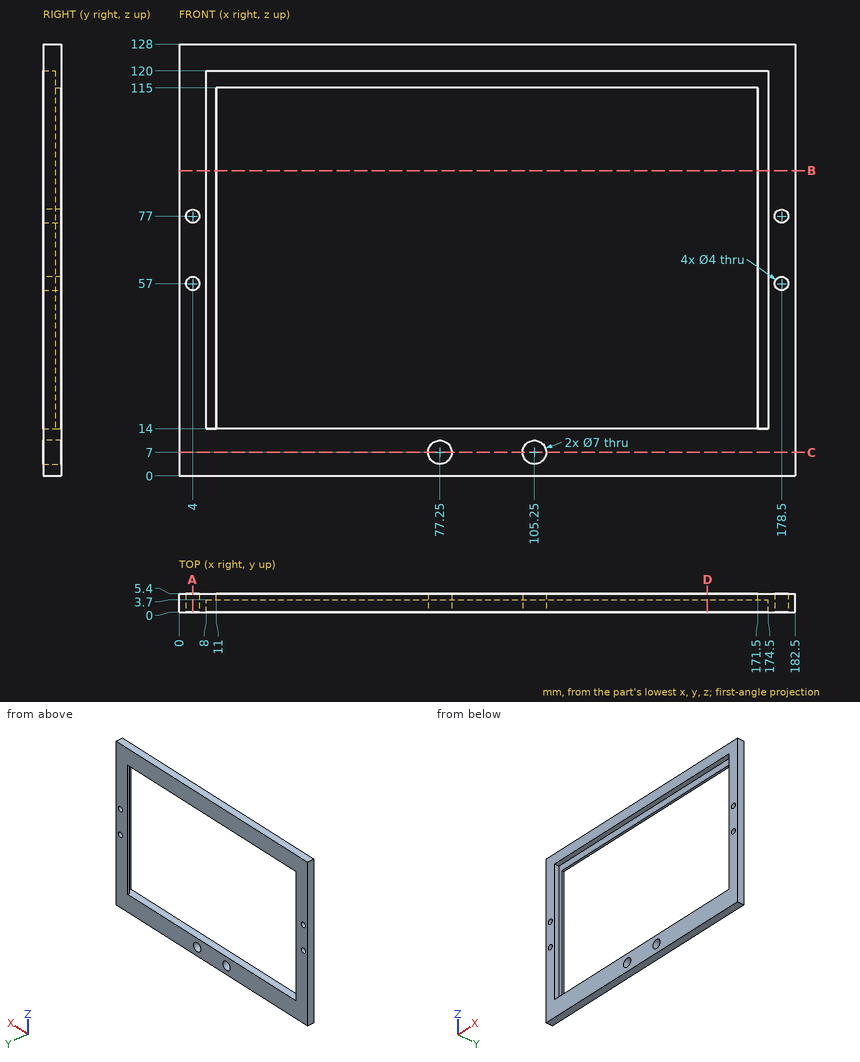
Design review of the part shown in the three views and the two pictorial views. Dimensions are in mm from the part's minimum x, y and z. Give positions to 0.01 mm unless a question says otherwise; leave off trailing zeros. Loops run counter-clockwise (first coordinate to the right, second up) from the corner with the lowest first, then second, coordinate; pieces in that order, holes last. Notation, with made-up numbers: (76.5, -20) -> (100.5, -20) arc R25 ccw to (100.5, 11) -> close; hole circle Ø8 at (56.5, 34). An arc over 180 degrees is marked (long way). Answer as a JSON object with one key per item and string values. Group by question number.
Q1. Take a section at A-A (x = 4). Write out the cut boundary in (y, z), plus the area to 3 significant figures.
Q2. Insertion check: pin 1 (6.5 mm diameter, centred on x = 105.25, z = 7, fed in from -Y). The pin has a flat end and moves straight along its axis. Give the tip position at first contact, or say it passes through.
Q3. Take a section at B-B (z = 90.5). Write out the cut boundary in (x, y), plus the area to 3 significant figures.
Q4. Take a section at D-D (x = 156.5). Write out the cut boundary in (y, z), plus the area to 3 significant figures.
Q5. Take a section at C-C (z = 7). Write out the cut boundary in (x, y), plus the area to 3 significant figures.
Q6. Wall thickness on line 1 along Z through (x, y) = (178.5, 2.9); line 2 along X through (y, z) = (4.2, 7); line 3 along X through (y, z) = (3.15, 77): over which ranges is each line inside the solid? List them lowest first.
Answer below:
{
 "1": {"outline": "(0, 0) -> (5.4, 0) -> (5.4, 55) -> (0, 55) -> close; (0, 59) -> (5.4, 59) -> (5.4, 75) -> (0, 75) -> close; (0, 79) -> (5.4, 79) -> (5.4, 128) -> (0, 128) -> close", "area": "648 mm2"},
 "2": {"pin 1": "passes through"},
 "3": {"outline": "(0, 0) -> (8, 0) -> (8, 3.7) -> (11, 3.7) -> (11, 5.4) -> (0, 5.4) -> close; (171.5, 3.7) -> (174.5, 3.7) -> (174.5, 0) -> (182.5, 0) -> (182.5, 5.4) -> (171.5, 5.4) -> close", "area": "96.6 mm2"},
 "4": {"outline": "(0, 0) -> (5.4, 0) -> (5.4, 14) -> (0, 14) -> close; (0, 120) -> (3.7, 120) -> (3.7, 115) -> (5.4, 115) -> (5.4, 128) -> (0, 128) -> close", "area": "127 mm2"},
 "5": {"outline": "(0, 0) -> (73.75, 0) -> (73.75, 5.4) -> (0, 5.4) -> close; (80.75, 0) -> (101.75, 0) -> (101.75, 5.4) -> (80.75, 5.4) -> close; (108.75, 0) -> (182.5, 0) -> (182.5, 5.4) -> (108.75, 5.4) -> close", "area": "910 mm2"},
 "6": {"line 1": "z = 0 to 55, 59 to 75, 79 to 128", "line 2": "x = 0 to 73.75, 80.75 to 101.75, 108.75 to 182.5", "line 3": "x = 0 to 2, 6 to 8, 174.5 to 176.5, 180.5 to 182.5"}
}
